```python
from build123d import *

# Parameters (mm, degrees)
SKETCH_281X300_25_R   = 2.15
SKETCH_281X300_25_R_2 = 2.2
SKETCH_281X300_25_R_3 = 1.6
F_4MM_DEPTH           = 4
FILLET_1_R            = 8


with BuildPart() as part:
    # Sketch 281x300__25 → 4mm (new body)
    with BuildSketch(Plane.XY):
        Polygon((-55.5, 150), (-55.5, 57), (-130.5, 57), (-130.5, -57), (-55.5, -57), (-55.5, -150), (57.5, -150), (57.5, -57), (128.5, -57), (128.5, 57), (57.5, 57), (57.5, 150), align=None)
        with Locations((-45, 140)):
            Circle(SKETCH_281X300_25_R, mode=Mode.SUBTRACT)
        with Locations((26, -140)):
            Circle(SKETCH_281X300_25_R_2, mode=Mode.SUBTRACT)
        with Locations((-24, -140)):
            Circle(SKETCH_281X300_25_R_2, mode=Mode.SUBTRACT)
        with Locations((118.5, 10)):
            Circle(SKETCH_281X300_25_R_3, mode=Mode.SUBTRACT)
        with Locations((118.5, -10)):
            Circle(SKETCH_281X300_25_R_3, mode=Mode.SUBTRACT)
        with Locations((-120.5, 10)):
            Circle(SKETCH_281X300_25_R_3, mode=Mode.SUBTRACT)
        with Locations((-120.5, -10)):
            Circle(SKETCH_281X300_25_R_3, mode=Mode.SUBTRACT)
        with Locations((118.5, 43)):
            Circle(SKETCH_281X300_25_R_3, mode=Mode.SUBTRACT)
        with Locations((118.5, -43)):
            Circle(SKETCH_281X300_25_R_3, mode=Mode.SUBTRACT)
        with Locations((-120.5, 43)):
            Circle(SKETCH_281X300_25_R_3, mode=Mode.SUBTRACT)
        with Locations((-120.5, -43)):
            Circle(SKETCH_281X300_25_R_3, mode=Mode.SUBTRACT)
        with Locations((47, 140)):
            Circle(SKETCH_281X300_25_R, mode=Mode.SUBTRACT)
        with Locations((-45, -140)):
            Circle(SKETCH_281X300_25_R, mode=Mode.SUBTRACT)
        with Locations((47, -140)):
            Circle(SKETCH_281X300_25_R, mode=Mode.SUBTRACT)
    extrude(amount=F_4MM_DEPTH)

    # Fillet 1
    fillet_1_edges = [part.edges().sort_by_distance(p)[0] for p in [
        (-130.5, 57, 2),
        (-55.5, 57, 2),
        (-55.5, 150, 2),
        (57.5, 150, 2),
        (57.5, 57, 2),
        (128.5, 57, 2),
        (128.5, -57, 2),
        (57.5, -57, 2),
        (57.5, -150, 2),
        (-55.5, -150, 2),
        (-55.5, -57, 2),
        (-130.5, -57, 2),
    ]]
    fillet(fillet_1_edges, radius=FILLET_1_R)


solid = part.part
```
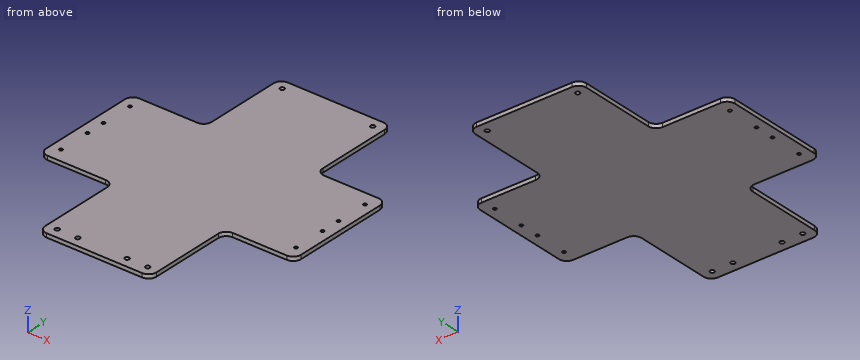
Geometry: final body of the model. Coordinates: model frame, mm. Coordinates: 2 decimals unless noted, no trailing zeros. Order: outer loops, then holes, each group sorted by start corner. A loop starts at its lowest first (then second) coordinate and runs counter-clockwise, first axis right, second up. Notation, with made-up numbers: M 47,16 L 59,16 A30 ccw 59,39 Z; hole C 7.5,-18.5 d9. An arc over 180 degrees is marked long. Answer as CSV lines item,"result".
Q1. First-contact query: P1, Ø2, axis at x = 90, z = 1.5, coming from the -Y side; P2, Ø2, axis at y = -100.5, z = 2.5, coming from the -X side; P3, Ø2, axis at y = -102, z = 1.5, coming from the +X side. Flat tips, straight axial feed; report the tip coordinate or a pass-through.
Answers:
P1,"stops at y = -57"
P2,"stops at x = -55.5"
P3,"stops at x = 57.5"
Q2. Section B-B on y = 89.5. Return the cut outline in (x, z), and give its area (3 significant figures).
Answers:
outline,"M -55.5,0 L 57.5,0 L 57.5,4 L -55.5,4 Z"
area,"452 mm^2"
Q3. Line query: probe 1 along Y at (x, z) = (-120.5, 1.5); probe 2 along Y at (x, z) = (118, 2.2); probe 3 along Y at (x, z) = (-100, 2.9). Output: solid intervals per line, ascending. Write a range as [from, to].
Answers:
probe 1,"y = [-57, -44.6], [-41.4, -11.6], [-8.4, 8.4], [11.6, 41.4], [44.6, 57]"
probe 2,"y = [-57, -44.52], [-41.48, -11.52], [-8.48, 8.48], [11.52, 41.48], [44.52, 57]"
probe 3,"y = [-57, 57]"
Q4. Section A-A on x = -71. Return the cut outline in (y, z).
Answers:
outline,"M -57,0 L 57,0 L 57,4 L -57,4 Z"
Q5. Section C-C on z = 2.1. Count the separate pieces of the cut face and the enclosed holes in it, and give its area (3 significant figures).
Answers:
separate pieces,"1"
enclosed holes,"14"
area,"50,300 mm^2"
